from build123d import *

# Parameters (mm, degrees)
F1_DEPTH  = 3.81
F3_DEPTH  = 5.461
F5_R      = 1.27
F6_DEPTH  = 9.272
F7_W      = 17.78
F7_H      = 11.43
F8_DEPTH  = 84.3534
F8_TAPER  = -5
F9_R      = 4.088765
F10_DEPTH = 93.6254001
F10_TAPER = -2.9356734464
F11_W     = 32.5399324597
F11_H     = 26.1899324597
F12_DEPTH = 15.24
F14_D     = 19.939
F14_DEPTH = 20.066
F14_TIP   = 5.9902799414


with BuildPart() as f1:
    # F0 (on Top) → F1 (new body)
    with BuildSketch(Plane.XY):
        with BuildLine():
            Line((4.1806183802, 5.7049052394), (-3.0799473447, 5.7049052394))
            ThreePointArc((-3.0799473447, 5.7049052394), (-12.6238, 0), (-3.0799473447, -5.7049052394))
            Line((-3.0799473447, -5.7049052394), (4.1806183802, -5.7049052394))
            ThreePointArc((4.1806183802, -5.7049052394), (11.8491, 0), (4.1806183802, 5.7049052394))
        make_face()
    extrude(amount=-F1_DEPTH)

    # F2 (on Top) → F3 (join)
    with BuildSketch(Plane.XY):
        with BuildLine():
            ThreePointArc((-10.8865895661, 4.4142863374), (-12.6238, 0), (-10.8865895661, -4.4142863374))
            ThreePointArc((-10.8865895661, -4.4142863374), (11.7475, 0), (-10.8865895661, 4.4142863374))
        make_face()
    extrude(amount=F3_DEPTH)

    # F5 (on face) → F6 (cut, through all)
    with BuildSketch(Plane.XY.offset(5.461)):
        with Locations((0, -7.62)):
            Circle(F5_R)
        with Locations((0, 7.62)):
            Circle(F5_R)
    extrude(amount=-F6_DEPTH, mode=Mode.SUBTRACT)

    # F7 (on face) → F8 (join)
    with BuildSketch(Plane.XY.offset(5.461)):
        Rectangle(F7_W, F7_H)
    extrude(amount=F8_DEPTH, taper=F8_TAPER)

    # F9 (on face) → F10 (cut, through all)
    with BuildSketch(Plane(origin=(0, 0, -3.81), x_dir=(1, 0, 0), z_dir=(0, 0, -1))):
        Circle(F9_R)
    extrude(amount=-F10_DEPTH, taper=F10_TAPER, mode=Mode.SUBTRACT)

    # F11 (on face) → F12 (join)
    with BuildSketch(Plane.XY.offset(89.8144)):
        Rectangle(F11_W, F11_H)
    extrude(amount=F12_DEPTH)

    # F14
    with Locations(Plane.XY.offset(105.0544)):
        with Locations((0, 0)):
            Hole(F14_D / 2, depth=F14_DEPTH)
            with Locations((0, 0, -(F14_DEPTH + F14_TIP / 2))):  # 118° drill point
                Cone(0, F14_D / 2, F14_TIP, mode=Mode.SUBTRACT)


solid = f1.part
Model file for the job. Use its own axes, mm. A direction names the side the tool comes from. Round coordinates to 2 decimals unless told otherwise and drop trailing zeros.
1. Drop flat-ended pins along their axis: P1, Ø6, axis at x = 7, z = 69, coming from the +Y side; P2, Ø3, axis at x = 2, y = 9, coming from the -Z side; P3, Ø3, axis at x = -0.5, z = -2, coming from the +Y side. Give the stop position or say it passes through.
Check values:
P1: stops at y = 11.54
P2: stops at z = 0
P3: stops at y = 5.7
2. Wall check: probe 1 along Y at (x, z) = (0, 2.7); probe 2 along X at (y, z) = (0, 98); probe 3 along Y at (x, z) = (0, 1). Give the ranges that are in metal, low to high.
Check values:
probe 1: y = -11.75 to -8.89, -6.35 to -4.42, 4.42 to 6.35, 8.89 to 11.75
probe 2: x = -16.27 to -9.97, 9.97 to 16.27
probe 3: y = -11.75 to -8.89, -6.35 to -4.34, 4.34 to 6.35, 8.89 to 11.75
3. Tool access for faces 5 (the flat face through (1, 5.705, -2)), 6 (the flat face through (0, -5.705, -2)), 7 (the cylindrical face through (-5.36, 8.406, 94.881)), 8 (the flat face through (0, -13.095, 97)), 9 (the cylindrical face through (-0.28, -8.86, 2.77)): list every direction of +Z, -Z, +X, -X, +Y, -Y with a clear straight run to the whole face (end or side of a thin tool).
Check values:
face 5: -Z, +Y
face 6: -Z, -Y
face 7: +Z
face 8: +Z, -Z, +X, -X, -Y
face 9: -Z
4. Mould opens along X. For faces 1 (the flat face through (-16.27, 0, 97)), 2 (the cylindrical face through (11.847, -0.155, -1.878)), 3 (the flat face through (0, 13.095, 97)), 4 (the cylindrical face through (11.74, -0.45, 2.69)) say: +X half, -X half, draft (parallel to the pull), parting line (faces both ways), or undercut.
Check values:
face 1: -X half
face 2: undercut
face 3: draft
face 4: parting line
5. Band-saw the part on A-A, the plane x = 0. Count the separate pieces of the cut face and the enclosed holes in it, and give its area (3 significant figures).
Check values:
separate pieces: 4
enclosed holes: 0
area: 598 mm2
